Part model, mm, in its own coordinate system. A direction names the side the tool comes from. Coordinates: 2 decimals unless noted, no trailing zeros. Loops run counter-clockwise (first coordinate to the right, second up) from the corner with the lowest first, then second, coordinate; pieces in that order, holes last. Notation, with made-up numbers: M 65.5,-23 L 89.5,-23 A24 ccw 89.5,8 Z; hole C 21,-15 d8. An arc over 180 degrees is marked long. Use a Markdown table: item, result. Add a question column.
1) Wall check: probe 1 along X at (y, z) = (-9, 4); probe 2 along X at (y, z) = (12, 4.5); probe 3 along X at (y, z) = (-2, 1.25). Give the ranges that are in metal, low to high. Write a range as from..to.
2) Pull direction Y, two halves, no side cores. Call faces 6 (the flat face through (2.57, 23.41, 0.88)), 7 (the flat face through (1.8, -7.3, 0)), 8 (the cylindrical face through (10.352, -0.131, 2.958)): released by +Y, released by -Y, zero draft, split by the parting line, or undercut.
3) Tool access for faces 1 (the flat face through (-22.176, -16.275, 3.625)), 2 (the flat face through (-22.2, -15.4, 1.52)), 3 (the flat face through (18.998, -13.89, 5.146)), 4 (the flat face through (-21.76, 9.75, 5.15)), 5 (the flat face through (22.94, 10.89, 0.88)): list every direction of +Z, -Z, +X, -X, +Y, -Y with a clear straight run to the whole face (end or side of a thin tool).
4) Pin check, flat tips, straight feed: pin 1 Ø5 at (x, y) = (-7.18, 12.43) entering from -Z; pin 2 Ø1.5 at (y, z) = (5.5, 3) entering from -X; pin 3 Ø1 at (x, y) = (-5.5, 17.5) entering from +Z; pin 4 Ø14.5 at (x, y) = (0, 0) entering from +Z (3 decimals). Stop position of each tip, or through.
5) Band-saw the part on B-B (y = 28). List the corners of the cut face in (x, z), plus the area to 3 significant figures.
6) Band-saw the part on A-A (y = 0). List the corners of the cut face in (x, z), plus the area to 3 significant figures.
from build123d import *

# Parameters (mm, degrees)
F0_R         = 6.35
F1_DEPTH     = 6
F2_C1_SIZE2  = 3
F2_C1_SIZE   = 1.7320508076
F2_C2_SIZE2  = 3
F2_C2_SIZE   = 1.7320508076
F2_C3_SIZE2  = 3
F2_C3_SIZE   = 1.7320508076
F2_C4_SIZE2  = 3
F2_C4_SIZE   = 1.7320508076
F2_C5_SIZE2  = 1.7320508076
F2_C5_SIZE   = 3
F2_C6_SIZE2  = 3
F2_C6_SIZE   = 1.7320508076
F2_C7_SIZE2  = 3
F2_C7_SIZE   = 1.7320508076
F2_C8_SIZE2  = 3
F2_C8_SIZE   = 1.7320508076
F2_C9_SIZE2  = 1.7320508076
F2_C9_SIZE   = 3
F2_C10_SIZE2 = 3
F2_C10_SIZE  = 1.7320508076
F2_C11_SIZE2 = 1.7320508076
F2_C11_SIZE  = 3
F2_C12_SIZE2 = 3
F2_C12_SIZE  = 1.7320508076
F2_C13_SIZE2 = 1.7320508076
F2_C13_SIZE  = 3
F2_C14_SIZE2 = 3
F2_C14_SIZE  = 1.7320508076
F2_C15_SIZE2 = 3
F2_C15_SIZE  = 1.7320508076
F2_C16_SIZE2 = 3
F2_C16_SIZE  = 1.7320508076
F2_C17_SIZE2 = 1.7320508076
F2_C17_SIZE  = 3
F2_C18_SIZE2 = 3
F2_C18_SIZE  = 1.7320508076
F2_C19_SIZE2 = 3
F2_C19_SIZE  = 1.7320508076
F2_C20_SIZE2 = 3
F2_C20_SIZE  = 1.7320508076
F2_C21_SIZE2 = 1.7320508076
F2_C21_SIZE  = 3
F2_C22_SIZE2 = 3
F2_C22_SIZE  = 1.7320508076
F2_C23_SIZE2 = 3
F2_C23_SIZE  = 1.7320508076
F2_C24_SIZE2 = 3
F2_C24_SIZE  = 1.7320508076
F3_R         = 1


with BuildPart() as f1:
    # F0 (on Top) → F1 (new body)
    with BuildSketch(Plane.XY):
        with BuildLine():
            Line((6.0983324846, 16.2798387553), (0, 38.1))
            Line((0, 38.1), (-6.0983324846, 16.2798387553))
            ThreePointArc((-6.0983324846, 16.2798387553), (-5.175, 8.9633629292), (-11.0495876893, 13.42123023))
            Line((-11.0495876893, 13.42123023), (-32.9955678842, 19.05))
            Line((-32.9955678842, 19.05), (-17.1479201739, 2.8586085253))
            ThreePointArc((-17.1479201739, 2.8586085253), (-10.35, 0), (-17.1479201739, -2.8586085253))
            Line((-17.1479201739, -2.8586085253), (-32.9955678842, -19.05))
            Line((-32.9955678842, -19.05), (-11.0495876893, -13.42123023))
            ThreePointArc((-11.0495876893, -13.42123023), (-5.175, -8.9633629292), (-6.0983324846, -16.2798387553))
            Line((-6.0983324846, -16.2798387553), (0, -38.1))
            Line((0, -38.1), (6.0983324846, -16.2798387553))
            ThreePointArc((6.0983324846, -16.2798387553), (5.175, -8.9633629292), (11.0495876893, -13.42123023))
            Line((11.0495876893, -13.42123023), (32.9955678842, -19.05))
            Line((32.9955678842, -19.05), (17.1479201739, -2.8586085253))
            ThreePointArc((17.1479201739, -2.8586085253), (10.35, 0), (17.1479201739, 2.8586085253))
            Line((17.1479201739, 2.8586085253), (32.9955678842, 19.05))
            Line((32.9955678842, 19.05), (11.0495876893, 13.42123023))
            ThreePointArc((11.0495876893, 13.42123023), (5.175, 8.9633629292), (6.0983324846, 16.2798387553))
        make_face()
        Circle(F0_R, mode=Mode.SUBTRACT)
    extrude(amount=F1_DEPTH)

    # F2: chamfer of 3 x 1.7320508076 on 24 edges, made by hand

    # F2_c1
    f2_c1_edges = [f1.edges().sort_by_distance(p)[0] for p in [
        (22.0225777867, -16.235615115, 0),
    ]]
    f2_c1_side = f1.faces().sort_by_distance((22.0225777867, -16.235615115, 0.0346410162))[0]
    chamfer(f2_c1_edges, length=F2_C1_SIZE, length2=F2_C1_SIZE2, reference=f2_c1_side)

    # F2_c2
    f2_c2_edges = [f1.edges().sort_by_distance(p)[0] for p in [
        (22.0225777867, -16.235615115, 6),
    ]]
    f2_c2_side = f1.faces().sort_by_distance((22.0225777867, -16.235615115, 5.9653589838))[0]
    chamfer(f2_c2_edges, length=F2_C2_SIZE, length2=F2_C2_SIZE2, reference=f2_c2_side)

    # F2_c3
    f2_c3_edges = [f1.edges().sort_by_distance(p)[0] for p in [
        (23.0480423242, -8.8867074098, 0),
    ]]
    f2_c3_side = f1.faces().sort_by_distance((23.0232860482, -8.9109381093, 0))[0]
    chamfer(f2_c3_edges, length=F2_C3_SIZE, length2=F2_C3_SIZE2, reference=f2_c3_side)

    # F2_c4
    f2_c4_edges = [f1.edges().sort_by_distance(p)[0] for p in [
        (23.0480423242, -8.8867074098, 6),
    ]]
    f2_c4_side = f1.faces().sort_by_distance((23.0480423242, -8.8867074098, 5.9653589838))[0]
    chamfer(f2_c4_edges, length=F2_C4_SIZE, length2=F2_C4_SIZE2, reference=f2_c4_side)

    # F2_c5
    f2_c5_edges = [f1.edges().sort_by_distance(p)[0] for p in [
        (25.071744029, 10.9543042626, 0),
    ]]
    f2_c5_side = f1.faces().sort_by_distance((25.046987753, 10.9785349621, 0))[0]
    chamfer(f2_c5_edges, length=F2_C5_SIZE, length2=F2_C5_SIZE2, reference=f2_c5_side)

    # F2_c6
    f2_c6_edges = [f1.edges().sort_by_distance(p)[0] for p in [
        (25.071744029, 10.9543042626, 6),
    ]]
    f2_c6_side = f1.faces().sort_by_distance((25.071744029, 10.9543042626, 5.9653589838))[0]
    chamfer(f2_c6_edges, length=F2_C6_SIZE, length2=F2_C6_SIZE2, reference=f2_c6_side)

    # F2_c7
    f2_c7_edges = [f1.edges().sort_by_distance(p)[0] for p in [
        (19.220135535, 15.5168364554, 0),
    ]]
    f2_c7_side = f1.faces().sort_by_distance((19.2287417983, 15.4832815417, 0))[0]
    chamfer(f2_c7_edges, length=F2_C7_SIZE, length2=F2_C7_SIZE2, reference=f2_c7_side)

    # F2_c8
    f2_c8_edges = [f1.edges().sort_by_distance(p)[0] for p in [
        (19.220135535, 15.5168364554, 6),
    ]]
    f2_c8_side = f1.faces().sort_by_distance((19.220135535, 15.5168364554, 5.9653589838))[0]
    chamfer(f2_c8_edges, length=F2_C8_SIZE, length2=F2_C8_SIZE2, reference=f2_c8_side)

    # F2_c9
    f2_c9_edges = [f1.edges().sort_by_distance(p)[0] for p in [
        (3.0491662423, 27.1899193776, 0),
    ]]
    f2_c9_side = f1.faces().sort_by_distance((3.015803703, 27.1805951634, 0))[0]
    chamfer(f2_c9_edges, length=F2_C9_SIZE, length2=F2_C9_SIZE2, reference=f2_c9_side)

    # F2_c10
    f2_c10_edges = [f1.edges().sort_by_distance(p)[0] for p in [
        (3.0491662423, 27.1899193776, 6),
    ]]
    f2_c10_side = f1.faces().sort_by_distance((3.0491662423, 27.1899193776, 5.9653589838))[0]
    chamfer(f2_c10_edges, length=F2_C10_SIZE, length2=F2_C10_SIZE2, reference=f2_c10_side)

    # F2_c11
    f2_c11_edges = [f1.edges().sort_by_distance(p)[0] for p in [
        (-3.8279067892, 24.4035438652, 0),
    ]]
    f2_c11_side = f1.faces().sort_by_distance((-3.7945442499, 24.394219651, 0))[0]
    chamfer(f2_c11_edges, length=F2_C11_SIZE, length2=F2_C11_SIZE2, reference=f2_c11_side)

    # F2_c12
    f2_c12_edges = [f1.edges().sort_by_distance(p)[0] for p in [
        (-3.8279067892, 24.4035438652, 6),
    ]]
    f2_c12_side = f1.faces().sort_by_distance((-3.8279067892, 24.4035438652, 5.9653589838))[0]
    chamfer(f2_c12_edges, length=F2_C12_SIZE, length2=F2_C12_SIZE2, reference=f2_c12_side)

    # F2_c13
    f2_c13_edges = [f1.edges().sort_by_distance(p)[0] for p in [
        (-22.0225777867, 16.235615115, 0),
    ]]
    f2_c13_side = f1.faces().sort_by_distance((-22.03118405, 16.2020602013, 0))[0]
    chamfer(f2_c13_edges, length=F2_C13_SIZE, length2=F2_C13_SIZE2, reference=f2_c13_side)

    # F2_c14
    f2_c14_edges = [f1.edges().sort_by_distance(p)[0] for p in [
        (-22.0225777867, 16.235615115, 6),
    ]]
    f2_c14_side = f1.faces().sort_by_distance((-22.0225777867, 16.235615115, 5.9653589838))[0]
    chamfer(f2_c14_edges, length=F2_C14_SIZE, length2=F2_C14_SIZE2, reference=f2_c14_side)

    # F2_c15
    f2_c15_edges = [f1.edges().sort_by_distance(p)[0] for p in [
        (-23.0480423242, 8.8867074098, 0),
    ]]
    f2_c15_side = f1.faces().sort_by_distance((-23.0232860482, 8.9109381093, 0))[0]
    chamfer(f2_c15_edges, length=F2_C15_SIZE, length2=F2_C15_SIZE2, reference=f2_c15_side)

    # F2_c16
    f2_c16_edges = [f1.edges().sort_by_distance(p)[0] for p in [
        (-23.0480423242, 8.8867074098, 6),
    ]]
    f2_c16_side = f1.faces().sort_by_distance((-23.0480423242, 8.8867074098, 5.9653589838))[0]
    chamfer(f2_c16_edges, length=F2_C16_SIZE, length2=F2_C16_SIZE2, reference=f2_c16_side)

    # F2_c17
    f2_c17_edges = [f1.edges().sort_by_distance(p)[0] for p in [
        (-25.071744029, -10.9543042626, 0),
    ]]
    f2_c17_side = f1.faces().sort_by_distance((-25.046987753, -10.9785349621, 0))[0]
    chamfer(f2_c17_edges, length=F2_C17_SIZE, length2=F2_C17_SIZE2, reference=f2_c17_side)

    # F2_c18
    f2_c18_edges = [f1.edges().sort_by_distance(p)[0] for p in [
        (-25.071744029, -10.9543042626, 6),
    ]]
    f2_c18_side = f1.faces().sort_by_distance((-25.071744029, -10.9543042626, 5.9653589838))[0]
    chamfer(f2_c18_edges, length=F2_C18_SIZE, length2=F2_C18_SIZE2, reference=f2_c18_side)

    # F2_c19
    f2_c19_edges = [f1.edges().sort_by_distance(p)[0] for p in [
        (-19.220135535, -15.5168364554, 0),
    ]]
    f2_c19_side = f1.faces().sort_by_distance((-19.2287417983, -15.4832815417, 0))[0]
    chamfer(f2_c19_edges, length=F2_C19_SIZE, length2=F2_C19_SIZE2, reference=f2_c19_side)

    # F2_c20
    f2_c20_edges = [f1.edges().sort_by_distance(p)[0] for p in [
        (-19.220135535, -15.5168364554, 6),
    ]]
    f2_c20_side = f1.faces().sort_by_distance((-19.220135535, -15.5168364554, 5.9653589838))[0]
    chamfer(f2_c20_edges, length=F2_C20_SIZE, length2=F2_C20_SIZE2, reference=f2_c20_side)

    # F2_c21
    f2_c21_edges = [f1.edges().sort_by_distance(p)[0] for p in [
        (-3.0491662423, -27.1899193776, 0),
    ]]
    f2_c21_side = f1.faces().sort_by_distance((-3.015803703, -27.1805951634, 0))[0]
    chamfer(f2_c21_edges, length=F2_C21_SIZE, length2=F2_C21_SIZE2, reference=f2_c21_side)

    # F2_c22
    f2_c22_edges = [f1.edges().sort_by_distance(p)[0] for p in [
        (-3.0491662423, -27.1899193776, 6),
    ]]
    f2_c22_side = f1.faces().sort_by_distance((-3.0491662423, -27.1899193776, 5.9653589838))[0]
    chamfer(f2_c22_edges, length=F2_C22_SIZE, length2=F2_C22_SIZE2, reference=f2_c22_side)

    # F2_c23
    f2_c23_edges = [f1.edges().sort_by_distance(p)[0] for p in [
        (3.8279067892, -24.4035438652, 0),
    ]]
    f2_c23_side = f1.faces().sort_by_distance((3.7945442499, -24.394219651, 0))[0]
    chamfer(f2_c23_edges, length=F2_C23_SIZE, length2=F2_C23_SIZE2, reference=f2_c23_side)

    # F2_c24
    f2_c24_edges = [f1.edges().sort_by_distance(p)[0] for p in [
        (3.8279067892, -24.4035438652, 6),
    ]]
    f2_c24_side = f1.faces().sort_by_distance((3.8279067892, -24.4035438652, 5.9653589838))[0]
    chamfer(f2_c24_edges, length=F2_C24_SIZE, length2=F2_C24_SIZE2, reference=f2_c24_side)

    # F3
    f3_edges = [f1.edges().sort_by_distance(p)[0] for p in [
        (-6.35, 0, 0),
        (-6.35, 0, 6),
    ]]
    fillet(f3_edges, radius=F3_R)


solid = f1.part
Entries:
| question | item | result |
|---|---|---|
| 1 | probe 1 | -23.16..-9.24, -5.11..5.11, 9.24..23.16 |
| 1 | probe 2 | -25.53..-11.15, -3.2..3.2, 11.15..25.53 |
| 1 | probe 3 | -10.89..-6.03, 6.03..10.89 |
| 2 | face 6 | released by +Y |
| 2 | face 7 | zero draft |
| 2 | face 8 | undercut |
| 3 | face 1 | +Z, -Z, -Y |
| 3 | face 2 | -Z, -Y |
| 3 | face 3 | +Z, -Y |
| 3 | face 4 | +Z, -X |
| 3 | face 5 | -Z, +X |
| 4 | pin 1 | through |
| 4 | pin 2 | x = -20.47 |
| 4 | pin 3 | z = 4.7 |
| 4 | pin 4 | z = 5.995 |
| 5 | outline | M -2.82,1.73 L 0,0.16 L 2.82,1.73 L 2.82,4.27 L 0,5.84 L -2.82,4.27 Z |
| 5 | area | 23.2 mm2 |
| 6 | outline | M -10.35,0 L -7.35,0 A1 ccw -6.35,1 L -6.35,5 A1 ccw -7.35,6 L -10.35,6 Z; M 6.35,1 A1 ccw 7.35,0 L 10.35,0 L 10.35,6 L 7.35,6 A1 ccw 6.35,5 Z |
| 6 | area | 47.1 mm2 |
